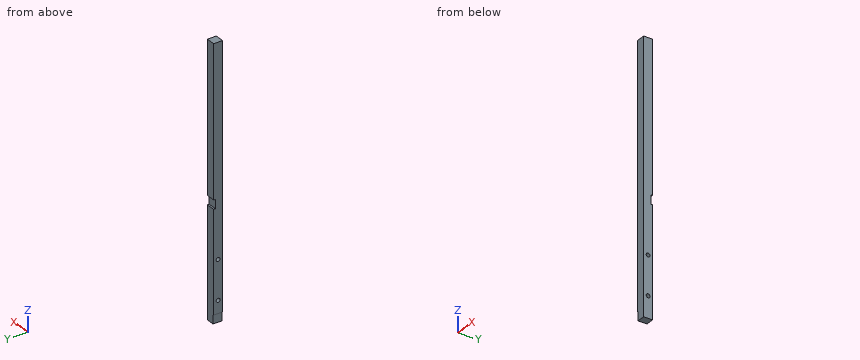
```python
from build123d import *

# Parameters (mm, degrees)
BOSS_EXTRU_1_START      = 7
ESQUISSE1_W             = 10
ESQUISSE1_H             = 10
BOSS_EXTRU_1_DEPTH      = 300
ESQUISSE4_W             = 10
ESQUISSE4_H             = 2
ENL_V_MAT_EXTRU_3_DEPTH = 11
ESQUISSE6_W             = 10
ESQUISSE6_H             = 10
ENL_V_MAT_EXTRU_5_DEPTH = 1
D_GAGEMENT_M41_D        = 4.3


with BuildPart() as part:
    # Esquisse1 → Boss.-Extru.1 (new body)
    with BuildSketch(Plane.XY.offset(BOSS_EXTRU_1_START)):
        Rectangle(ESQUISSE1_W, ESQUISSE1_H)
    extrude(amount=BOSS_EXTRU_1_DEPTH)

    # Esquisse4 → Enlèv. mat.-Extru.3 (cut, through all)
    with BuildSketch(Plane(origin=(5, 0, 0), x_dir=(0, 0, -1), z_dir=(1, 0, 0))):
        with Locations((-135, 4)):
            Rectangle(ESQUISSE4_W, ESQUISSE4_H)
    extrude(amount=-ENL_V_MAT_EXTRU_3_DEPTH, mode=Mode.SUBTRACT)

    # Esquisse6 → Enlèv. mat.-Extru.5 (cut)
    with BuildSketch(Plane.ZY.offset(5)):
        with Locations((12, 0)):
            Rectangle(ESQUISSE6_W, ESQUISSE6_H)
    extrude(amount=-ENL_V_MAT_EXTRU_5_DEPTH, mode=Mode.SUBTRACT)

    # Dégagement M41 (through all)
    with Locations(Plane.ZY.offset(5)):
        with Locations((74.69, 0), (31.09, 0)):
            Hole(D_GAGEMENT_M41_D / 2)


solid = part.part
```
Here's how the part is built. I have some questions about the finished solid (model axes, mm). Give positions to 0.01 mm unless a question says otherwise; leave off trailing zeros. Write each loop counter-clockwise with the first axis right and the second up, starting at its lowest first coordinate (ties: lowest second). Pieces come first, ordered by that corner, then holes. Notation, with made-up numbers: M 73.5,-21.5 L 123.5,-21.5 A17 cw 123.5,-15.5 Z; hole C 68,-37 d2. An arc over 180 degrees is marked long. Put each result on its own line as item: value. Start each with the question number.
Item 1: If we section it at B-B, the plane x = -1.25: Write out the boundary of the cut face in (y, z).
Item 2: Will these pins go through, and if not, where does the flat tip stop? pin 1 (3 mm diameter, centred on y = 1, z = 14, fed in from -X); pin 2 (3 mm diameter, centred on x = -1, z = 134, fed in from +Y).
Item 3: If we section it at A-A, the plane y = 0: Write out the boundary of the cut face in (x, z).
Item 4: I need wall thicknesses on L1, parallel to Z at x = 2, y = 0.5; L2, parallel to Z at x = -1.25, y = 0.75; L3, parallel to Y at x = -0.5, z = 31.09. Which ranges of each line are inside material? Lowest first, please. Write a range as from..to.
Values:
1. outline: M -5,7 L 5,7 L 5,130 L 3,130 L 3,140 L 5,140 L 5,307 L -5,307 Z; hole C 0,31.09 d4.3; hole C 0,74.69 d4.3
2. pin 1: x = -4
2. pin 2: y = 3
3. outline: M -5,17 L -4,17 L -4,7 L 5,7 L 5,28.94 L -5,28.94 Z; M -5,33.24 L 5,33.24 L 5,72.54 L -5,72.54 Z; M -5,76.84 L 5,76.84 L 5,307 L -5,307 Z
4. L1: 7..29, 33.18..72.6, 76.78..307
4. L2: 7..29.08, 33.1..72.68, 76.7..307
4. L3: -5..-2.15, 2.15..5
